Answer from the drawing. Dimensions are ordinates in mm from the lowest x, y and z of the part. A direction names the side the tool comes from. Give positions to 0.01 mm unless a question says otherwise; leave off trailing zeros. Write each loop counter-clockwise with the first axis right and the second up, starting at its lowest first coordinate (ties: lowest second). Pieces come first, ordered by that corner, then holes.
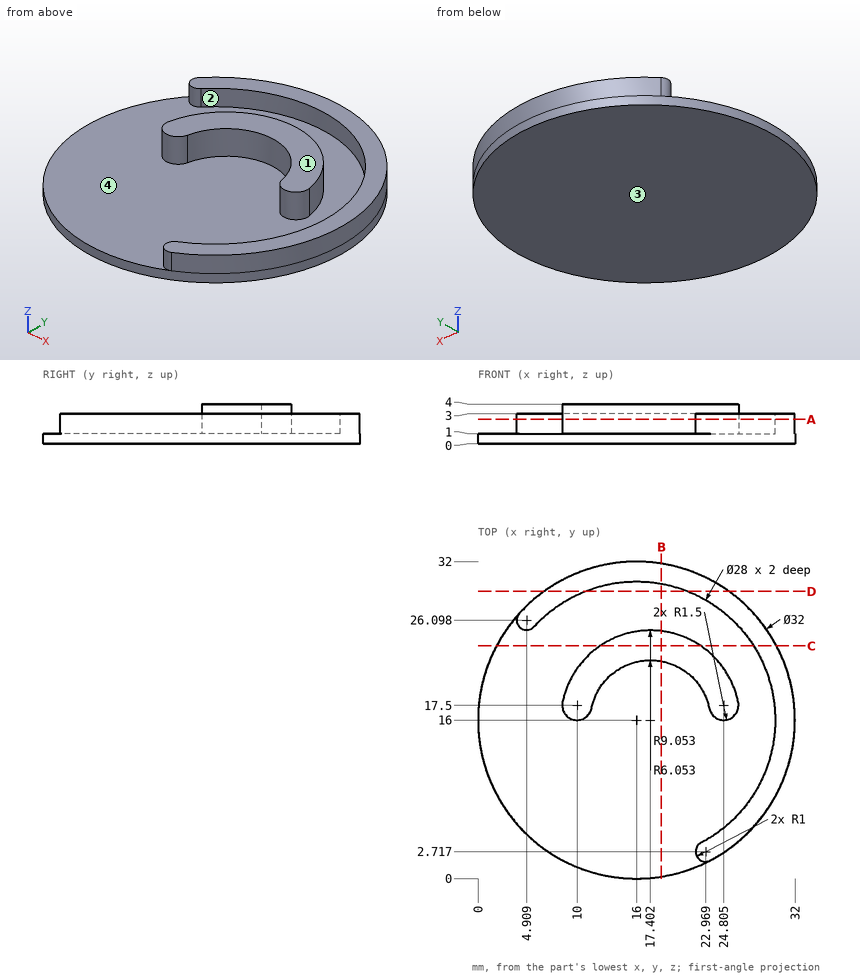
Item 1: A cutting plane is placed at D-D, the plane y = 29. Give the vertices of the cut face in (x, z).
Conclusion:
outline: (6.67, 0) - (25.33, 0) - (25.33, 3) - (21.2, 3) - (21.2, 1) - (10.8, 1) - (10.8, 3) - (6.67, 3) - close
Item 2: Which of the six approach directions +Z, -Z, +X, -X, +Y, -Y give full straight-line access (tool end or side, diameter ignored) to the marked faces 3 and 4?
Conclusion:
face 3: -Z, +X, -X, +Y, -Y
face 4: +Z
Item 3: A cutting plane is placed at B-B, the plane x = 18.5. Give the vertices of the cut face in (y, z) (1 decimal).
Conclusion:
outline: (0.2, 0) - (31.8, 0) - (31.8, 3) - (29.8, 3) - (29.8, 1) - (25, 1) - (25, 4) - (22, 4) - (22, 1) - (0.2, 1) - close
Item 4: Determine the mould class of the marked faces 1 and 2 for opening direction Y: pulls with the +Y half, pulls with the -Y half, needs draft (parallel to the pull), parting line crosses it, or undercut.
Conclusion:
face 1: needs draft
face 2: undercut
Item 5: Each of these flat-tipped pins is pushed along its axis until it touches: P1, Ø1, axis at x = 4.5, z = 2, coming from the +Y side; P2, Ø8.5, axis at x = 16, y = 17, coming from the +Z side; P3, Ø1.5, axis at x = 25, z = 1.5, coming from the -Y side. Where does it stop, or does it pass through?
Conclusion:
P1: stops at y = 27.62
P2: stops at z = 1
P3: stops at y = 2.29
Item 6: A cutting plane is placed at C-C, the plane y = 23.5. Give the vertices of the cut face in (x, z).
Conclusion:
outline: (1.87, 0) - (30.13, 0) - (30.13, 3) - (27.82, 3) - (27.82, 1) - (22.47, 1) - (22.47, 4) - (12.33, 4) - (12.33, 1) - (1.87, 1) - close
Item 7: A cutting plane is placed at A-A, the plane z = 2.45. Give the vertices of the cut face in (x, y) (1 decimal).
Conclusion:
outline: (4.2, 26.8) arc R1 ccw to (5.6, 25.4) arc R14 cw (long way) to (22.5, 3.6) arc R1 ccw to (23.4, 1.8) arc R16 ccw (long way) to start; (8.5, 17.8) arc R1.5 ccw to (11.5, 17.2) arc R6.1 cw to (23.3, 17.2) arc R1.5 ccw to (26.3, 17.8) arc R9.1 ccw to start
Item 8: Consider probe 1 along Z at (x, y) = (15, 25.5); probe 2 along Y at (x, z) = (19, 1.4) (1 decimal); probe 3 along Y at (x, z) = (16, 2.3). Determine where each line is inside the solid, lowest interval first.
Conclusion:
probe 1: z = 0 to 1
probe 2: y = 21.8 to 24.9, 29.7 to 31.7
probe 3: y = 21.89 to 24.94, 30 to 32
